The listing builds one solid part. Answer for the finished solid, in the listing's coordinates (mm). A direction names the side the tool comes from. Coordinates: 2 decimals unless noted, no trailing zeros. Loops run counter-clockwise (first coordinate to the right, second up) from the corner with the lowest first, then second, coordinate; pieces in that order, holes last. Notation, with made-up numbers: M 55,69 L 71,69 A29 ccw 71,93 Z; hole C 8,-10.5 d11. An arc over 180 degrees is marked long. Return JSON: item names as keys, results as strings. Group by question number.
1. Section C-C (z = 4.3) is taken. Write down the section's boundary in (x, y).
2. Given P1, Ø1.5, axis at y = 48.5, z = 3.5, coming from the +X side; P2, Ø1.5, axis at x = -3, z = 3.5, coming from the -Y side; P3, Ø1.5, axis at y = 40.5, z = 3.5, coming from the -X side; P4, Ø6.5, axis at x = 9.8, y = 23, coming from the +Z side, each flat-ended and moving along its own axis, determine where each tip first touches the part or whether it passes through.
3. Section B-B (x = 23) is taken. Write down the section's boundary in (y, z), then the cut area to 3 significant figures.
4. Straight lines are drawn through the part: L1, parallel to Y at x = 9.8, z = 1.65; L2, parallel to X at y = 22, z = 2.85; L3, parallel to Y at x = 23.5, z = 1. For each, find the intervals that lie inside material, in ascending order. Write a range as from..to.
5. The mould has two halves that part along Y. Classify faces 5 (the face through (23, -5, 2)), 6 (the face through (21.63, 33.41, 2.46)), 7 (the face through (23, 51, 2)), 8 (the face through (30.5, -3, 2)): pulls with the +Y half, pulls with the -Y half, needs draft (parallel to the pull), parting line crosses it, or undercut.
6. Section D-D (y = 32.5) is taken. Write down the section's boundary in (x, z), then the cut area to 3 significant figures.
7. Which of the six approach directions +Z, -Z, +X, -X, +Y, -Y give full straight-line access (tool end or side, diameter ignored) to faces 1 (the face through (48, 15.5, 2)), 2 (the face through (18, 49, 2)), 3 (the face through (28, 48, 2)), 4 (the face through (-3, 15.5, 2))?
8. Section A-A (y = 23) is taken. Write down the section's boundary in (x, z), then the cut area to 3 significant figures.
```python
from build123d import *

# Parameters (mm, degrees)
F1_R     = 2.1
F1_R_2   = 10.5
F2_DEPTH = 5


with BuildPart() as f2:
    # F1 (on Top) → F2 (new body)
    with BuildSketch(Plane.XY):
        Polygon((0, 15.5), (0, 0), (15.5, 0), (15.5, -5), (30.5, -5), (30.5, 0), (46, 0), (46, 15.5), (51, 15.5), (51, 30.5), (46, 30.5), (46, 46), (28, 46), (28, 51), (18, 51), (18, 46), (0, 46), (0, 30.5), (-5, 30.5), (-5, 15.5), align=None)
        with Locations((9.8, 23)):
            Circle(F1_R, mode=Mode.SUBTRACT)
        with Locations((23, 23)):
            Circle(F1_R_2, mode=Mode.SUBTRACT)
        with Locations((36.2, 23)):
            Circle(F1_R, mode=Mode.SUBTRACT)
    extrude(amount=F2_DEPTH)


solid = f2.part
```
Worked out:
{
 "1": {"outline": "M -5,15.5 L 0,15.5 L 0,0 L 15.5,0 L 15.5,-5 L 30.5,-5 L 30.5,0 L 46,0 L 46,15.5 L 51,15.5 L 51,30.5 L 46,30.5 L 46,46 L 28,46 L 28,51 L 18,51 L 18,46 L 0,46 L 0,30.5 L -5,30.5 Z; hole C 9.8,23 d4.2; hole C 23,23 d21; hole C 36.2,23 d4.2"},
 "2": {"P1": "x = 28", "P2": "y = 15.5", "P3": "x = 0", "P4": "z = 5"},
 "3": {"outline": "M -5,0 L 12.5,0 L 12.5,5 L -5,5 Z; M 33.5,0 L 51,0 L 51,5 L 33.5,5 Z", "area": "175 mm^2"},
 "4": {"L1": "0..20.9, 25.1..46", "L2": "-5..7.95, 11.65..12.55, 33.45..34.35, 38.05..51", "L3": "-5..12.51, 33.49..51"},
 "5": {"face 5": "pulls with the -Y half", "face 6": "undercut", "face 7": "pulls with the +Y half", "face 8": "needs draft"},
 "6": {"outline": "M 0,0 L 18.53,0 L 18.53,5 L 0,5 Z; M 27.47,0 L 46,0 L 46,5 L 27.47,5 Z", "area": "185 mm^2"},
 "7": {"face 1": "+Z, -Z, +X, -Y", "face 2": "+Z, -Z, -X, +Y", "face 3": "+Z, -Z, +X, +Y", "face 4": "+Z, -Z, -X, -Y"},
 "8": {"outline": "M -5,0 L 7.7,0 L 7.7,5 L -5,5 Z; M 11.9,0 L 12.5,0 L 12.5,5 L 11.9,5 Z; M 33.5,0 L 34.1,0 L 34.1,5 L 33.5,5 Z; M 38.3,0 L 51,0 L 51,5 L 38.3,5 Z", "area": "133 mm^2"}
}
